Job drawing, mm, ordinate dimensions from the low corner. One solid piece. A direction names the side the tool comes from. Give positions to 0.01 mm unless a question says otherwise; leave off trailing zeros. Loops run counter-clockwise (first coordinate to the right, second up) from the corner with the lowest first, then second, coordinate; pieces in that order, holes last. Notation, with made-up numbers: (46, 2.5) - (54, 2.5) arc R26 cw to (54, 26.5) - close; hole circle Ø6 at (34.5, -38). An arc over 180 degrees is marked (long way). Answer as CSV lines item,"result". Start each with the question number.
Item 1: Drill centre lines: L1, parallel to Y at x = 61, z = 1; L2, parallel to Z at x = 78, y = 10.5. Where is each one in solid material? Low to high. Write a range as from..to.
Item 2: Tool access for the marked faces 1 and 2: list every direction of +Z, -Z, +X, -X, +Y, -Y with a clear straight run to the whole face (end or side of a thin tool).
Item 3: Saw through at A-A on x = 31. Give the cut face in (y, z), plus the area to 3 significant figures.
Item 4: Saw through at C-C on y = 10. Give the cut face in (x, z).
Item 5: Pin check, flat tips, straight feed: pin 1 (5.5 mm diameter, centred on x = 61, y = 10, fed in from +Z); pin 2 (3.5 mm diameter, centred on x = 31, y = 10, fed in from +Z); pin 3 (10 mm diameter, centred on x = 48, y = 2, fed in from -Z); pin 4 (1.5 mm diameter, centred on x = 32.5, z = 6.5, fed in from +Y). Stop position of each tip, or through.
Item 6: Saw through at D-D on x = 76. Give the cut face in (y, z), plus the area to 3 significant figures.
Item 7: Saw through at B-B on z = 14. Give the cut face in (x, y), plus the area to 3 significant figures.
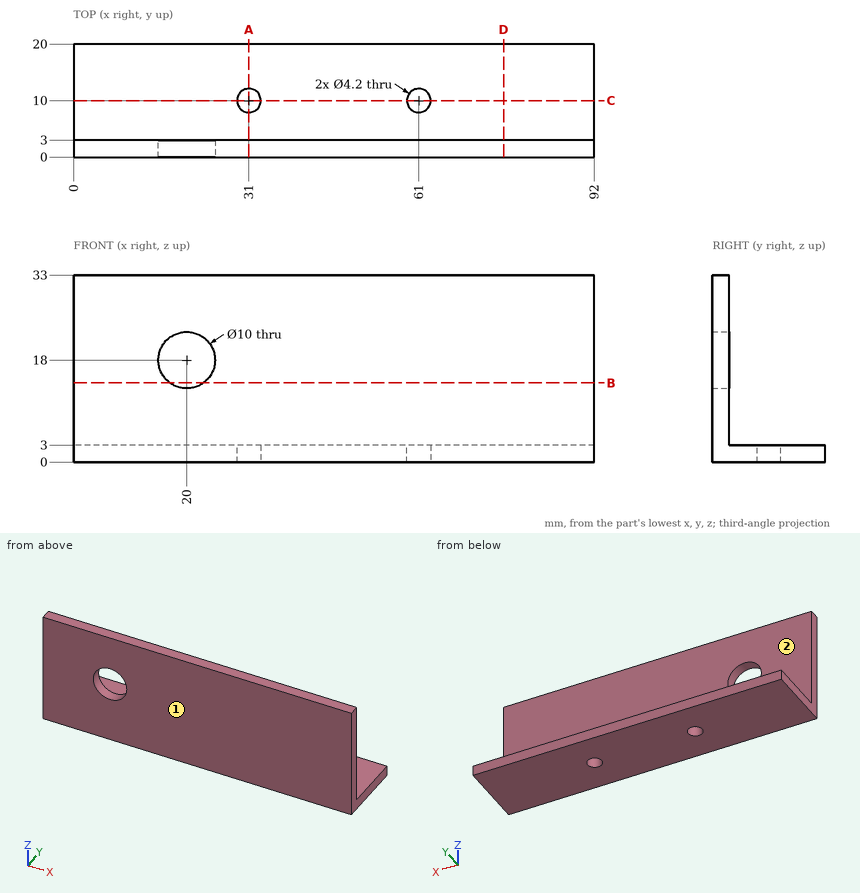
Responses:
1,L1,"0..7.9, 12.1..20"
1,L2,"0..3"
2,face 1,"+Z, -Z, +X, -X, -Y"
2,face 2,"+Z, +X, -X, +Y"
3,outline,"(0, 0) - (7.9, 0) - (7.9, 3) - (3, 3) - (3, 33) - (0, 33) - close; (12.1, 0) - (20, 0) - (20, 3) - (12.1, 3) - close"
3,area,"137 mm2"
4,outline,"(0, 0) - (28.9, 0) - (28.9, 3) - (0, 3) - close; (33.1, 0) - (58.9, 0) - (58.9, 3) - (33.1, 3) - close; (63.1, 0) - (92, 0) - (92, 3) - (63.1, 3) - close"
5,pin 1,"z = 3"
5,pin 2,"through"
5,pin 3,"z = 0"
5,pin 4,"y = 3"
6,outline,"(0, 0) - (20, 0) - (20, 3) - (3, 3) - (3, 33) - (0, 33) - close"
6,area,"150 mm2"
7,outline,"(0, 0) - (17, 0) - (17, 3) - (0, 3) - close; (23, 0) - (92, 0) - (92, 3) - (23, 3) - close"
7,area,"258 mm2"
